```python
from build123d import *

# Parameters (mm, degrees)
F0_R            = 20
F1_DEPTH        = 5
F3_D            = 3.3
F3_COPIES_COUNT = 4
F5_D            = 6.05


# Not quite as in the source:
# - a pattern or mirror of a feature is missing from the dataset's text; its kind, count and spacing are read off the source's solid


with BuildPart() as f1:
    # F0 (on Top) → F1 (new body)
    with BuildSketch(Plane.XY):
        Circle(F0_R)
    extrude(amount=F1_DEPTH)

    # F3 (through all)
    with Locations(Plane.XY.offset(5)):
        with Locations((0, 12)):
            f3 = Hole(F3_D / 2)

    # F3_copies: F3 ×4 about axis
    f3_copies_axis = Axis((0, 0, 0), (0, 0, 1))
    for i in range(1, F3_COPIES_COUNT):
        add(f3.rotate(f3_copies_axis, i * 360 / F3_COPIES_COUNT), mode=Mode.SUBTRACT)

    # F5 (through all)
    with Locations(Plane.XY.offset(5)):
        with Locations((0, 0)):
            Hole(F5_D / 2)


solid = f1.part
```
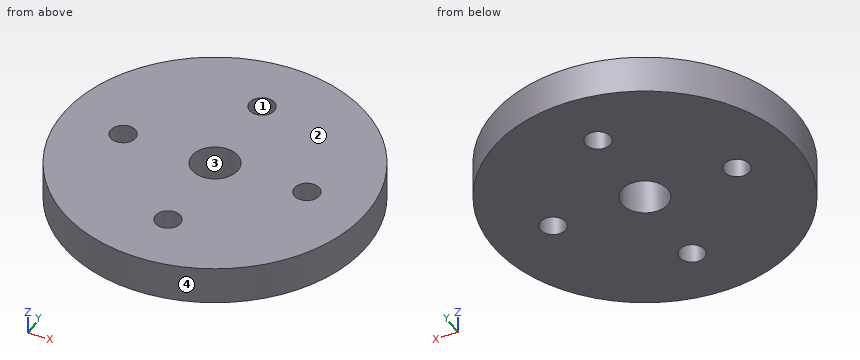
The model under review builds one solid part; all positions refer to its coordinate system, in mm. Face numbers are marked on the shaded views. Coordinates: 2 decimals unless noted, no trailing zeros. Write each loop counter-clockwise with the first axis right and the second up, starting at its lowest first coordinate (ties: lowest second). Pieces come first, ordered by that corner, then holes. Notation, with made-up numbers: (-40, 0) - (-18, 0) arc R33 cw to (-18, 35) - close; hole circle Ø8 at (42, 89). An arc over 180 degrees is marked (long way). Write item = value, one per line.
(1) Consider section C-C, the plane z = 3.8. Give the boundary of the cut face in (x, y) (3 decimals).
Result sheet:
outline = circle Ø40 at (0, 0); hole circle Ø3.3 at (-12, 0); hole circle Ø6.05 at (0, 0); hole circle Ø3.3 at (0, -12); hole circle Ø3.3 at (0, 12); hole circle Ø3.3 at (12, 0)
(2) Consider section B-B, the plane x = -12. Give the boundary of the cut face in (y, z).
Result sheet:
outline = (-16, 0) - (-1.65, 0) - (-1.65, 5) - (-16, 5) - close; (1.65, 0) - (16, 0) - (16, 5) - (1.65, 5) - close
(3) For P1, Ø3, axis at y = -3.5, z = 3, coming from the -X side; P2, Ø1.5, axis at y = -12, z = 3, coming from the +X side; P3, Ø3, axis at y = 10.5, z = 4, coming from the -X side, all flat-tipped, find the tip position at first contact; note any pin that passes through.
Result sheet:
P1 = -19.9
P2 = 16.54
P3 = -17.86
(4) Consider section A-A, the plane y = 0. Give the boundary of the cut face in (x, z) (3 decimals).
Result sheet:
outline = (-20, 0) - (-13.65, 0) - (-13.65, 5) - (-20, 5) - close; (-10.35, 0) - (-3.025, 0) - (-3.025, 5) - (-10.35, 5) - close; (3.025, 0) - (10.35, 0) - (10.35, 5) - (3.025, 5) - close; (13.65, 0) - (20, 0) - (20, 5) - (13.65, 5) - close
(5) For line 1 (Y direction, x = 0, z = 1.9) (3 decimals); line 2 (X direction, y = 1.5, z = 2.65); line 3 (Y direction, x = -1, z = 4.35), list the stretches that pass through material, from the lowest coordinate up. Write a range as [from, to].
Result sheet:
line_1 = [-20, -13.65], [-10.35, -3.025], [3.025, 10.35], [13.65, 20]
line_2 = [-19.94, -12.69], [-11.31, -2.63], [2.63, 11.31], [12.69, 19.94]
line_3 = [-19.97, -13.31], [-10.69, -2.85], [2.85, 10.69], [13.31, 19.97]
(6) Mouldability with a two-part tool opening along Y and no side actions: class the marked faces 1, 2, 3 and 4 as pulls with the +Y half, pulls with the -Y half, needs draft (parallel to the pull), parting line crosses it, or undercut.
Result sheet:
face_1 = undercut
face_2 = needs draft
face_3 = undercut
face_4 = parting line crosses it
